Job drawing, mm, ordinate dimensions from the low corner. One solid piece. A direction names the side the tool comes from. Coordinates: 2 decimals unless noted, no trailing zeros. Write each loop counter-clockwise with the first axis right and the second up, starting at its lowest first coordinate (ties: lowest second). Pieces come first, ordered by that corner, then holes.
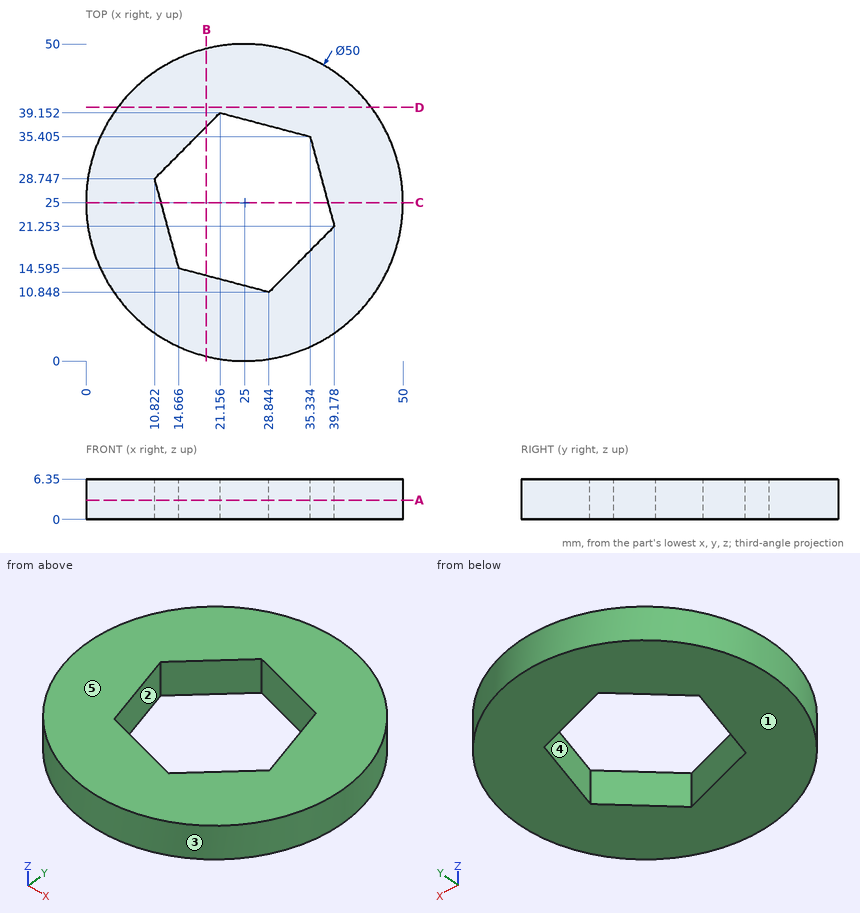
1. Saw through at B-B on x = 19. List the corners of the cut face in (y, z), plus the area to 3 significant figures.
Computed values:
outline: (0.73, 0) - (13.45, 0) - (13.45, 6.35) - (0.73, 6.35) - close; (36.98, 0) - (49.27, 0) - (49.27, 6.35) - (36.98, 6.35) - close
area: 159 mm2
2. 3-axis set-ups, long thin cutter, end or side, ignore diameter. For the marked faces 4 and 5: which of +Z, -Z, +X, -X, +Y, -Y reach the whole face in a straight line?
Computed values:
face 4: +Z, -Z
face 5: +Z, +X, -X, +Y, -Y
3. Probe line 1 along X through (y, z) = (30.5, 3) (1 decimal); line 2 along Y through (x, z) = (15.5, 2) (1 decimal); line 3 along Y through (x, z) = (20, 3) (1 decimal). List the from-to ranges inside material, lowest first.
Computed values:
line 1: x = 0.6 to 12.6, 36.7 to 49.4
line 2: y = 1.9 to 14.4, 33.5 to 48.1
line 3: y = 0.5 to 13.2, 38 to 49.5
4. Saw through at D-D on y = 40. List the corners of the cut face in (x, z), plus the area to 3 significant figures.
Computed values:
outline: (5, 0) - (45, 0) - (45, 6.35) - (5, 6.35) - close
area: 254 mm2
5. Saw through at C-C on y = 25. List the corners of the cut face in (x, z), plus the area to 3 significant figures.
Computed values:
outline: (0, 0) - (11.84, 0) - (11.84, 6.35) - (0, 6.35) - close; (38.16, 0) - (50, 0) - (50, 6.35) - (38.16, 6.35) - close
area: 150 mm2
6. Mould opens along Y. For the marked faces 1, 2 and 3 say: +Y half, -Y half, draft (parallel to the pull), parting line (faces both ways), or undercut.
Computed values:
face 1: draft
face 2: undercut
face 3: parting line
7. Flat gauge pin, fed straight in: pin 1 (2 mm diameter, centred on x = 30, z = 1.5, fed in from +Y). Where does the tip first touch, or does it go through?
Computed values:
pin 1: stops at y = 49.68
8. Saw through at A-A on z = 3. List the corners of the cut face in (x, y) (1 decimal), plus the area to 4 significant figures.
Computed values:
outline: circle Ø50 at (25, 25); hole (10.8, 28.7) - (14.7, 14.6) - (28.8, 10.8) - (39.2, 21.3) - (35.3, 35.4) - (21.2, 39.2) - close
area: 1,405 mm2
